Build history of the part. All positions in model axes, mm. A direction names the side the tool comes from. Give positions to 0.01 mm unless a question says otherwise; leave off trailing zeros. Write each loop counter-clockwise with the first axis right and the second up, starting at its lowest first coordinate (ties: lowest second). Pieces come first, ordered by that corner, then holes. Notation, with made-up numbers: M -6.75,40.5 L 10.25,40.5 A15 ccw 10.25,65.5 Z; hole C -28,52.25 d5. An arc over 180 degrees is marked long. One line per item, written item: value. Start each with the question number.
from build123d import *
from build123d.topology import SkipClean

# Parameters (mm, degrees)
SKETCH_1_R             = 5.5
EXTRUDE_1_DEPTH        = 68
CHAMFER_1_SIZE         = 0.5
SKETCH_2_R             = 4
EXTRUDE_2_DEPTH        = 8
CHAMFER_2_SIZE         = 0.5
HOLE_WIZARD_M5_1_D     = 4.2
HOLE_WIZARD_M5_1_DEPTH = 12.4
HOLE_WIZARD_M5_1_TIP   = 1.2618073
CHAMFER_3_SIZE         = 0.5
SKETCH_5_W             = 10
SKETCH_5_H             = 3
CUT_EXTRUDE_3_DEPTH    = 13


with BuildPart() as part:
    # 草图1 → 拉伸1 (new body)
    with BuildSketch(Plane.XY):
        Circle(SKETCH_1_R)
    extrude(amount=EXTRUDE_1_DEPTH)

    # 倒角1
    chamfer_1_edges = [part.edges().sort_by_distance(p)[0] for p in [
        (-5.5, 0, 0),
        (-5.5, 0, 68),
    ]]
    chamfer(chamfer_1_edges, length=CHAMFER_1_SIZE)

    # 草图2 → 拉伸2 (add)
    with BuildSketch(Plane.XY.offset(68)):
        Circle(SKETCH_2_R)
    extrude(amount=EXTRUDE_2_DEPTH)

    # 倒角2
    chamfer_2_edges = [part.edges().sort_by_distance(p)[0] for p in [
        (-4, 0, 76),
    ]]
    chamfer(chamfer_2_edges, length=CHAMFER_2_SIZE)

    # M5 螺纹孔1
    with Locations(Plane(origin=(0, 0, 0), x_dir=(-1, 0, 0), z_dir=(0, 0, -1))):
        with Locations((0, 0)):
            Hole(HOLE_WIZARD_M5_1_D / 2, depth=HOLE_WIZARD_M5_1_DEPTH)
            with Locations((0, 0, -(HOLE_WIZARD_M5_1_DEPTH + HOLE_WIZARD_M5_1_TIP / 2))):  # 118° drill point
                Cone(0, HOLE_WIZARD_M5_1_D / 2, HOLE_WIZARD_M5_1_TIP, mode=Mode.SUBTRACT)

    # 倒角3
    chamfer_3_edges = [part.edges().sort_by_distance(p)[0] for p in [
        (-2.1, 0, 0),
    ]]
    chamfer(chamfer_3_edges, length=CHAMFER_3_SIZE)

    # 草图5 → 拉伸3 (cut)
    with SkipClean():  # the faces are left unmerged after this step: merging them gives an invalid solid
        with BuildSketch(Plane.XY):
            with Locations((0, 6.5)):
                Rectangle(SKETCH_5_W, SKETCH_5_H)
        cut_extrude_3 = extrude(amount=CUT_EXTRUDE_3_DEPTH, mode=Mode.SUBTRACT)

    # 镜向1: 拉伸3 across plane
    add(cut_extrude_3.mirror(Plane.ZX), mode=Mode.SUBTRACT)


solid = part.part
1) Tool access for faces 1 (the face through (-0.867, -3.905, 71.698)), 2 (the face through (0, 0, 76)), 3 (the face through (0, -5, 6)), 4 (the face through (0, 5, 6)): list every direction of +Z, -Z, +X, -X, +Y, -Y with a clear straight run to the whole face (end or side of a thin tool).
2) Drop flat-ended pins along their axis: P1, Ø0.6, axis at x = -0.5, y = -5.5, coming from the -Z side; P2, Ø5, axis at x = -0.5, z = 9, coming from the -Y side; P3, Ø1.5, axis at x = -2.5, z = 62, coming from the -Y side. Give the stop position or say it passes through.
3) Probe line 1 along X through (y, z) = (0, 5.75); line 2 along Y through (x, z) = (0, 4); line 3 along Z through (x, y) = (-3.75, 1.5). List the from-to ranges inside material, lowest first. Write a range as from..to.
4) Mould opens along X. For faces 5 (the face through (2.003, 0.631, 6.533)), 6 (the face through (2, -2, 0)), 7 (the face through (-0.35, 0.11, 13.44)), 8 (the face through (5.08, -2.11, 33.53)) say: released by +X, released by -X, zero draft, split by the parting line, or undercut.
5) Band-saw the part on A-A (z = 8.5). List the corners of the cut face in (x, y), then the cut area to 3 significant figures.
6) Band-saw the part on B-B (z = 42). List the corners of the cut face in (x, y), then the cut area to 3 significant figures.
Model answer:
1. face 1: +Z
1. face 2: +Z, +X, -X, +Y, -Y
1. face 3: -Z, +X, -X, -Y
1. face 4: -Z, +X, -X, +Y
2. P1: stops at z = 13
2. P2: stops at y = -5
2. P3: stops at y = -5.21
3. line 1: x = -5.5..-2.1, 2.1..5.5
3. line 2: y = -5..-2.1, 2.1..5
3. line 3: z = 0..68
4. face 5: undercut
4. face 6: zero draft
4. face 7: undercut
4. face 8: split by the parting line
5. outline: M -2.29,-5 L 2.29,-5 A5.5 ccw 2.29,5 L -2.29,5 A5.5 ccw Z; hole C 0,0 d4.2
5. area: 78.1 mm²
6. outline: C 0,0 d11
6. area: 95.0 mm²
